```python
from build123d import *

# Parameters (mm, degrees)
F0_R     = 7.6453811345
F1_DEPTH = 25
F2_COUNT = 12


with BuildPart() as f1:
    # F0 (on Front) → F1 (new body)
    with BuildSketch(Plane.XZ):
        with BuildLine():
            ThreePointArc((-4.199583616, 26.5301707062), (0.2331271007, 26.859488305), (4.6594538037, 26.4532786342))
            ThreePointArc((4.6594538037, 26.4532786342), (4.5311676373, 28.7913934414), (3.9730198519, 31.0655326722))
            ThreePointArc((3.9730198519, 31.0655326722), (2.8779662016, 33.6301332845), (1.3244981356, 35.9459605158))
            ThreePointArc((1.3244981356, 35.9459605158), (0.0510003023, 34.8088199887), (-1.2719943746, 35.8879726168))
            ThreePointArc((-1.2719943746, 35.8879726168), (-2.7205256231, 33.5051012356), (-3.6999932599, 30.8941699945))
            ThreePointArc((-3.6999932599, 30.8941699945), (-4.1411626969, 28.7340788632), (-4.199583616, 26.5301707062))
        make_face()
        with BuildLine():
            ThreePointArc((-4.199583616, 26.5301707062), (-17.4453940129, -20.4241202499), (26.8605, 0))
            ThreePointArc((26.8605, 0), (20.5747626857, 17.2674723303), (4.6594538037, 26.4532786342))
            ThreePointArc((4.6594538037, 26.4532786342), (0.2331271007, 26.859488305), (-4.199583616, 26.5301707062))
        make_face()
        Circle(F0_R, mode=Mode.SUBTRACT)
    extrude(amount=F1_DEPTH)

    # F2: F1 ×12 about axis
    f2_axis = Axis((0, 0, 0), (0, 1, 0))


with BuildPart() as f1_1:
    add(f1.part)
    for i in range(1, F2_COUNT):
        add(f1.part.rotate(f2_axis, i * 360 / F2_COUNT))


solid = f1_1.part
```
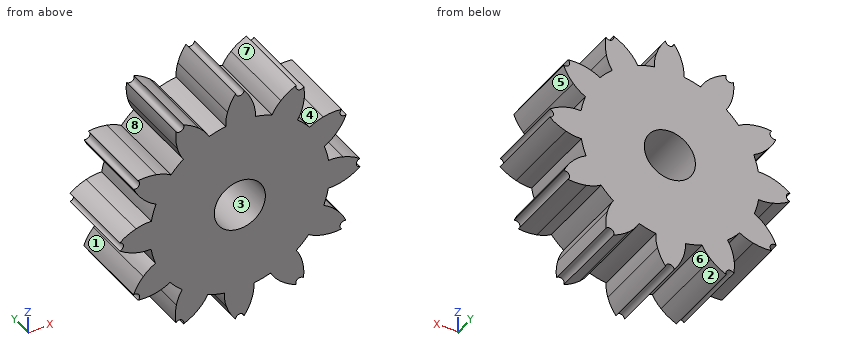
Geometry: final body of the model. Coordinates: model frame, mm. Face numbers are marked on the shaded views. A direction names the side the tool comes from. Coordinates: 2 decimals unless noted, no trailing zeros. Loops run counter-clockwise (first coordinate to the right, second up) from the corner with the lowest first, then second, coordinate; pieces in that order, holes last. Notation, with made-up numbers: (16.25, 39) -> (43.25, 39) arc R21 cw to (43.25, 54) -> close; hole circle Ø4 at (37, -39.75). An arc over 180 degrees is marked (long way). Use a Markdown table: item, result. Add a question column.
(1) Mould query, pull axis Z, two halves, no side actions, for the marked faces 6, 7 and 8. Classes: pulls with the +Z half, pulls with the -Z half, needs draft (parallel to the pull), parting line crosses it, or undercut.
(2) Access query for the marked faces 1, 2, 3, 4 and 5. Directions: +Z, -Z, +X, -X, +Y, -Y. A direction counts if a zero-diameter tool reaches every point of the face in a straight line with its end or side. Return the directions, or none.
(3) Line query: line 1 along X through (y, z) = (-11.5, 0); line 2 along X through (y, z) = (-22.5, -31.5). Output: solid intervals per line, ascending.
(4) Section query C-C, the plane z = 27.5. Return loops of the section in (x, y), plus the area to 3 significant figures.
(5) Section query A-A, the plane z = 0. Return loops of the section in (x, y).
(6) Pin query (flat end, axial travel): pin 1 Ø1 at (x, y) = (-27.5, -22.5) entering from +Z; pin 2 Ø12 at (y, z) = (-11.5, 16) entering from +X; pin 3 Ø9 at (x, z) = (0, 0) entering from +Y; pin 4 Ø8 at (y, z) = (-20, 11.5) entering from -X. Return the tip coordinate at first contact, or that it passes through.
(7) Section query B-B, the plane x = 0. Return loops of the section in (y, z).
Answer:
| question | item | result |
|---|---|---|
| 1 | face 6 | pulls with the -Z half |
| 1 | face 7 | pulls with the +Z half |
| 1 | face 8 | undercut |
| 2 | face 1 | -X, +Y, -Y |
| 2 | face 2 | -Z, +Y, -Y |
| 2 | face 3 | +Y, -Y |
| 2 | face 4 | +Z, +Y, -Y |
| 2 | face 5 | +X, +Y, -Y |
| 3 | line 1 | x = -34.81 to -7.65, 7.65 to 34.81 |
| 3 | line 2 | x = -16.79 to -16.37, -3.83 to 3.52, 16.11 to 16.74 |
| 4 | outline | (-19.1, -25) -> (-10.72, -25) -> (-10.72, 0) -> (-19.1, 0) -> close; (-4.22, -25) -> (4.66, -25) -> (4.66, 0) -> (-4.22, 0) -> close; (11.21, -25) -> (19.3, -25) -> (19.3, 0) -> (11.21, 0) -> close |
| 4 | area | 634 mm^2 |
| 5 | outline | (-34.81, -25) -> (-7.65, -25) -> (-7.65, 0) -> (-34.81, 0) -> close; (7.65, -25) -> (34.81, -25) -> (34.81, 0) -> (7.65, 0) -> close |
| 6 | pin 1 | stops at z = 19.31 |
| 6 | pin 2 | stops at x = 31.79 |
| 6 | pin 3 | passes through |
| 6 | pin 4 | stops at x = -31.05 |
| 7 | outline | (-25, -34.81) -> (0, -34.81) -> (0, -7.65) -> (-25, -7.65) -> close; (-25, 7.65) -> (0, 7.65) -> (0, 34.81) -> (-25, 34.81) -> close |
